The model under review builds one solid part; all positions refer to its coordinate system, in mm. Face numbers are marked on the shaded views. A direction names the side the tool comes from. Coordinates: 2 decimals unless noted, no trailing zeros. Loops run counter-clockwise (first coordinate to the right, second up) from the corner with the lowest first, then second, coordinate; pieces in that order, holes last. Notation, with made-up numbers: (-16, 69.5) - (43, 69.5) arc R16 ccw to (43, 87.5) - close; hole circle Ø10 at (-3, 16). An arc over 180 degrees is marked (long way). Answer in a Markdown table with one row per item. Add a question column.
(1) We need section B-B on y = 2.5. Give the number of separate pieces and of enclosed holes in the cut face, plus the area to 3 significant figures.
(2) For line 1 along Z through (x, y) = (-1.25, 9.25); line 2 along Z through (x, y) = (-0.5, 3.25); line 3 along X through (y, z) = (4.5, -10.5), list the stretches that pass through material, from the lowest coordinate up.
(3) Machinability: for the marked faces 1, 2 and 3, which of the approach directions +Z, -Z, +X, -X, +Y, -Y give a long, thin tool a straight path to every point of the face, cutting with its end or side? Answer none if there is none.
(4) We need section A-A on z = 0. Write out the cut boundary in (x, y), plus the area to 3 significant figures.
(5) Mouldability with a two-part tool opening along X and no side actions: class the marked faces 4, 5 and 6 as +X half, -X half, draft (parallel to the pull), parting line (faces both ways), or undercut.
(6) For P1, Ø5, axis at x = 3, z = -25.5, coming from the -Y side; P2, Ø2, axis at y = 6.5, z = 12, coming from the -X side; P3, Ø1, axis at x = -3.5, y = 3, coming from the -Z side, all flat-tipped, find the tip position at first contact; note any pin that passes through.
(7) We need section C-C on x = -2.75. Write out the cut boundary in (y, z).
Autodesk Inventor part; units mm, degrees
ref_plane "YZ Plane" through (0, 0, 0) normal (1, 0, 0) x (0, 1, 0)
ref_plane "XZ Plane" through (0, 0, 0) normal (0, 1, 0) x (-1, 0, 0)
ref_plane "XY Plane" through (0, 0, 0) normal (0, 0, 1) x (1, 0, 0)
sketch "Sketch1" plane through (0, 0, 0) normal (0, 1, 0) x (-1, 0, 0)
  circle A0 centre (0, 0) radius 2
  line L0 (0, 0) -> (0, -20) construction
  circle A1 centre (0, -20) radius 2
  arc A2 (0, -5) -> (0, 5) centre (0, 0) ccw
  arc A3 (0, -25) -> (0, -15) centre (0, -20) ccw
  line L1 (0, -5) -> (0, -15)
  line L2 (0, -10) -> (-5, -10) construction
  line L3 (-5, -10) -> (-5, -35) construction
  line L4 (-5, -10) -> (-5, 15) construction
  line L5 (0, 5) -> (0, 15)
  line L6 (0, 15) -> (-4, 15)
  line L7 (0, -25) -> (0, -35)
  line L8 (0, -35) -> (-4, -35)
  line L9 (-5, -10) -> (-5, 7.5)
  line L10 (-5, -10) -> (-5, -27.5)
  arc A4 (-4, 15) -> (-5, 7.5) centre (24.9994, 7.3167) ccw
  arc A5 (-5, -27.5) -> (-4, -35) centre (24.9994, -27.3167) ccw
  dimension "d0" = 4
  dimension "d1" = 20
  dimension "d2" = 4
  dimension "d3" = 10
  dimension "d4" = 10
  dimension "d5" = 5
  dimension "d6" = 25
  dimension "d7" = 25
  dimension "d8" = 10
  dimension "d9" = 4
  dimension "d10" = 10
  dimension "d11" = 4
  dimension "d12" = 17.5
  dimension "d13" = 17.5
  dimension "d14" = 30
  dimension "d15" = 30
extrude "Extrusion1" add sketch "Sketch1" along normal blind 10
fillet "Fillet1" radius 3 4 edges at (0, 5, 5) (0, 5, -5) (0, 5, -15) (0, 5, -25)
fillet "Fillet2" radius 1 4 edges at (0, 5, 15) (4, 5, 15) (0, 5, -35) (4, 5, -35)
fillet "Fillet3" radius 25 2 edges at (5, 5, 7.5) (5, 5, -27.5)
chamfer "Chamfer1" distance 0.25 angle 45 4 edges at (2, 10, -20) (2, 10, 0) (2, 0, 0) (2, 0, -20)
properties part number "Battery_Slide" material "Nylon 6/6"
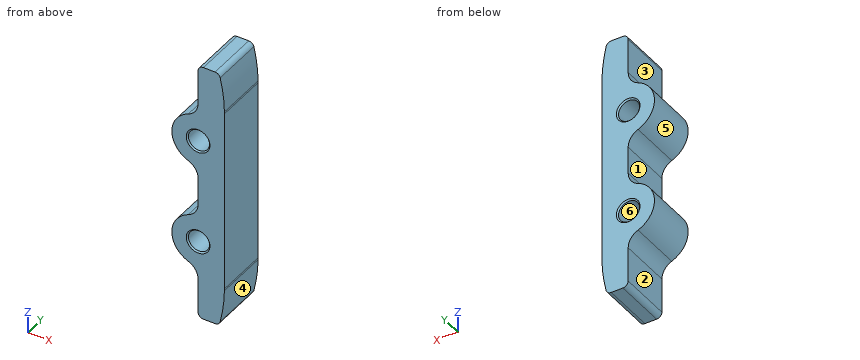
Outcome:
| question | item | result |
|---|---|---|
| 1 | separate pieces | 1 |
| 1 | enclosed holes | 2 |
| 1 | area | 302 mm² |
| 2 | line 1 | -24.98 to -21.56, -18.44 to -15.02, -4.98 to -1.56, 1.56 to 4.98 |
| 2 | line 2 | -25.76 to -21.94, -18.06 to -14.24, -5.76 to -1.94, 1.94 to 5.76 |
| 2 | line 3 | 0 to 5 |
| 3 | face 1 | -X, +Y, -Y |
| 3 | face 2 | -Z, -X, +Y, -Y |
| 3 | face 3 | +Z, -X, +Y, -Y |
| 4 | outline | (-5, 0) - (-2.25, 0) - (-2, 0.25) - (-2, 9.75) - (-2.25, 10) - (-5, 10) - close; (2, 0.25) - (2.25, 0) - (5, 0) - (5, 10) - (2.25, 10) - (2, 9.75) - close |
| 4 | area | 59.9 mm² |
| 5 | face 4 | +X half |
| 5 | face 5 | -X half |
| 5 | face 6 | undercut |
| 6 | P1 | y = 0 |
| 6 | P2 | x = 0 |
| 6 | P3 | z = -24 |
| 7 | outline | (0, -24.18) - (10, -24.18) - (10, -15.82) - (0, -15.82) - close; (0, -4.18) - (10, -4.18) - (10, 4.18) - (0, 4.18) - close |
